```python
from build123d import *

# Parameters (mm, degrees)
SKETCH1_R           = 32
BOSS_EXTRUDE1_DEPTH = 25
SKETCH2_R           = 22
BOSS_EXTRUDE2_DEPTH = 81
SKETCH3_R           = 12.5
BOSS_EXTRUDE3_DEPTH = 20
SKETCH4_R           = 16
CUT_EXTRUDE1_DEPTH  = 77
CUT_EXTRUDE2_DEPTH  = 145.899965493
CHAMFER1_SIZE       = 2.5
FILLET1_R           = 1


with BuildPart() as part:
    # Sketch1 → Boss-Extrude1 (new body)
    with BuildSketch(Plane.XY):
        Circle(SKETCH1_R)
    extrude(amount=BOSS_EXTRUDE1_DEPTH)

    # Sketch2 → Boss-Extrude2 (add)
    with BuildSketch(Plane.XY.offset(25)):
        Circle(SKETCH2_R)
    extrude(amount=BOSS_EXTRUDE2_DEPTH)

    # Sketch3 → Boss-Extrude3 (add)
    with BuildSketch(Plane.XY.offset(106)):
        Circle(SKETCH3_R)
    extrude(amount=BOSS_EXTRUDE3_DEPTH)

    # Sketch4 → Cut-Extrude1 (cut)
    with BuildSketch(Plane(origin=(0, 0, 0), x_dir=(-1, 0, 0), z_dir=(0, 0, -1))):
        Circle(SKETCH4_R)
    extrude(amount=-CUT_EXTRUDE1_DEPTH, mode=Mode.SUBTRACT)

    # Sketch5 → Cut-Extrude2 (cut, through all)
    with BuildSketch(Plane(origin=(0, 32, 0), x_dir=(1, 0, 0), z_dir=(0, 1, 0))):
        Polygon((3, -25), (3, -59), (-3, -58.60148044), (-3, -25), align=None)
    extrude(amount=-CUT_EXTRUDE2_DEPTH, mode=Mode.SUBTRACT)

    # Chamfer1
    chamfer1_edges = [part.edges().sort_by_distance(p)[0] for p in [
        (-12.5, 0, 126),
        (-32, 0, 0),
        (-32, 0, 25),
        (-22, 0, 106),
    ]]
    chamfer(chamfer1_edges, length=CHAMFER1_SIZE)

    # Fillet1
    fillet1_edges = [part.edges().sort_by_distance(p)[0] for p in [
        (-12.5, 0, 106),
        (-22, 0, 25),
        (16.583123952, 14.456832295, 25),
    ]]
    fillet(fillet1_edges, radius=FILLET1_R)


solid = part.part
```
The listing builds one solid part. Answer for the finished solid, in the listing's coordinates (mm). A direction names the side the tool comes from. Give positions to 0.01 mm unless a question says otherwise; leave off trailing zeros. Write each loop counter-clockwise with the first axis right and the second up, starting at its lowest first coordinate (ties: lowest second). Pieces come first, ordered by that corner, then holes. Notation, with made-up numbers: (-24, 37) - (14, 37) arc R18 cw to (14, 47) - close; hole circle Ø2 at (-0.5, 77.25). An arc over 180 degrees is marked (long way). Use one line per item in the form item = value. Start each with the question number.
1) Find section B-B on x = 0. Count the separate pieces of the cut face and the enclosed holes in it, plus the area to 3 significant figures.
2) Find section C-C on y = 0. Determine the outline of the cut face in (x, z).
3) The mould has two halves that part along X. Classify faces 1 (the face through (3.47, -15.62, 37.96)), 2 (the face through (13, -13, 0)), 3 (the face through (0, 18.9, 58.8)), 4 (the face through (-6.421, 28.917, 24.879)): pulls with the +X half, pulls with the -X half, needs draft (parallel to the pull), parting line crosses it, or undercut.
4) Find section D-D on z = 16.5. Determine the outline of the cut face in (x, y).
5) Consider line 1 along Y through (x, z) = (0, 19.5); line 2 along X through (y, z) = (-16, 34); line 3 along Z through (x, y) = (-5.5, 26). Determine where each line is inside the solid, lowest interval first. Write a range as from..to.
6) Flat-ended cylindrical pins translate along their axes: pin 1 Ø5.5 at (y, z) = (18, 41) entering from -X; pin 2 Ø5.5 at (y, z) = (18.5, 44.5) entering from +X; pin 3 Ø1.5 at (x, y) = (-15.5, -2.5) entering from +Z. Find the tip coordinate at first contact, or state that the pin passes through.
7) A tool of negligible diameter and unlimited length cuts with its end or side. For faces 5 (the face through (0, 0, 77)), 6 (the face through (0, 0, 126)), 7 (the face through (3, 19, 42)), 8 (the face through (13, 5, 106)), from which of +Z, -Z, +X, -X, +Y, -Y can it reach the whole face along a straight path? Write none if from no direction.
8) Find section A-A on z = 30. Determine the outline of the cut face in (x, y).
Geometry results:
q1.separate_pieces = 3
q1.enclosed_holes = 0
q1.area = 2,770 mm2
q2.outline = (-32, 2.5) - (-29.5, 0) - (-16, 0) - (-16, 77) - (16, 77) - (16, 0) - (29.5, 0) - (32, 2.5) - (32, 22.5) - (29.5, 25) - (23, 25) arc R1 cw to (22, 26) - (22, 103.5) - (19.5, 106) - (13.5, 106) arc R1 cw to (12.5, 107) - (12.5, 123.5) - (10, 126) - (-10, 126) - (-12.5, 123.5) - (-12.5, 107) arc R1 cw to (-13.5, 106) - (-19.5, 106) - (-22, 103.5) - (-22, 26) arc R1 cw to (-23, 25) - (-29.5, 25) - (-32, 22.5) - close
q3.face_1 = undercut
q3.face_2 = needs draft
q3.face_3 = undercut
q3.face_4 = parting line crosses it
q4.outline = circle Ø64 at (0, 0); hole circle Ø32 at (0, 0)
q5.line_1 = -32..-16, 16..32
q5.line_2 = -15.1..-3, 3..15.1
q5.line_3 = 0..25
q6.pin_1 = -15.86
q6.pin_2 = 15.36
q6.pin_3 = 106
q7.face_5 = -Z
q7.face_6 = +Z, +X, -X, +Y, -Y
q7.face_7 = +Y, -Y
q7.face_8 = +Z
q8.outline = (-3, -21.79) - (-3, -15.72) arc R16 cw to (-3, 15.72) - (-3, 21.79) arc R22 ccw to start; (3, -21.79) arc R22 ccw to (3, 21.79) - (3, 15.72) arc R16 cw to (3, -15.72) - close
